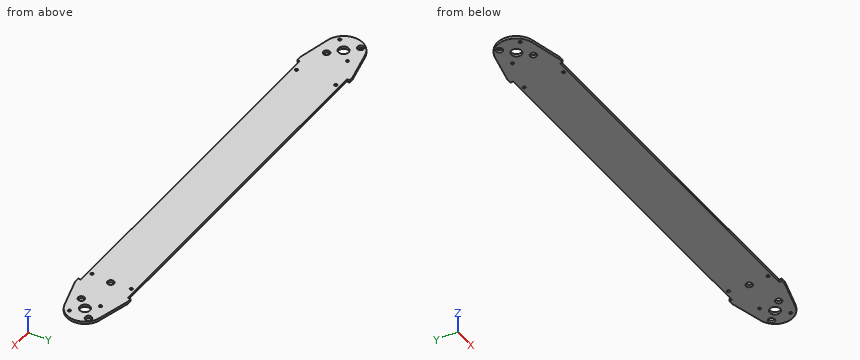
from build123d import *

# Parameters (mm, degrees)
F0_R     = 1.7272
F0_R_2   = 3.96875
F0_R_3   = 6.35
F1_DEPTH = 3.175


with BuildPart() as f1:
    # F0 (on Top) → F1 (new body)
    with BuildSketch(Plane.XY):
        with BuildLine():
            Line((-475.378193, 31.75), (-513.228467, 23.231407))
            ThreePointArc((-513.228467, 23.231407), (-531.812151, 0.128904), (-513.479674, -23.17344))
            Line((-513.479674, -23.17344), (-474.818103, -32.315493))
            Line((-474.818103, -32.315493), (-468.468103, -32.315493))
            Line((-468.468103, -32.315493), (-468.468103, -29.140493))
            Line((-468.468103, -29.140493), (-38.411718, -29.140493))
            Line((-38.411718, -29.140493), (-38.411718, -32.315493))
            Line((-38.411718, -32.315493), (-32.061718, -32.315493))
            Line((-32.061718, -32.315493), (6.126706, -21.36385))
            ThreePointArc((6.126706, -21.36385), (22.224151, 0.194294), (5.752253, 21.467701))
            Line((5.752253, 21.467701), (-32.621807, 31.75))
            Line((-32.621807, 31.75), (-38.971807, 31.75))
            Line((-38.971807, 31.75), (-38.971807, 28.575))
            Line((-38.971807, 28.575), (-469.028193, 28.575))
            Line((-469.028193, 28.575), (-469.028193, 31.75))
            Line((-469.028193, 31.75), (-475.378193, 31.75))
        make_face()
        with Locations((-454.180603, -24.377993)):
            Circle(F0_R, mode=Mode.SUBTRACT)
        with Locations((-520.909118, -12.909118)):
            Circle(F0_R, mode=Mode.SUBTRACT)
        with Locations((-495.090882, -12.909118)):
            Circle(F0_R_2, mode=Mode.SUBTRACT)
        with Locations((-52.699218, -24.377993)):
            Circle(F0_R, mode=Mode.SUBTRACT)
        with Locations((-11.786586, -11.786586)):
            Circle(F0_R_2, mode=Mode.SUBTRACT)
        with Locations((11.786586, -11.786586)):
            Circle(F0_R, mode=Mode.SUBTRACT)
        with Locations((-508, 0)):
            Circle(F0_R_3, mode=Mode.SUBTRACT)
        with Locations((-520.909118, 12.909118)):
            Circle(F0_R_2, mode=Mode.SUBTRACT)
        with Locations((-495.090882, 12.909118)):
            Circle(F0_R, mode=Mode.SUBTRACT)
        with Locations((-454.740693, 23.8125)):
            Circle(F0_R, mode=Mode.SUBTRACT)
        with Locations((-50.8, 0)):
            Circle(F0_R_2, mode=Mode.SUBTRACT)
        Circle(F0_R_3, mode=Mode.SUBTRACT)
        with Locations((-11.786586, 11.786586)):
            Circle(F0_R, mode=Mode.SUBTRACT)
        with Locations((11.786586, 11.786586)):
            Circle(F0_R_2, mode=Mode.SUBTRACT)
        with Locations((-53.259307, 23.8125)):
            Circle(F0_R, mode=Mode.SUBTRACT)
    extrude(amount=F1_DEPTH)


solid = f1.part
CAD build for the part. Positions are in the model's coordinates, mm. Give positions to 0.01 mm unless a question says otherwise; leave off trailing zeros. Order: outer loops, then holes, each group sorted by start corner. A loop starts at its lowest first (then second) coordinate and runs counter-clockwise, first axis right, second up. Notation, with made-up numbers: (11, 16) - (33, 16) arc R16 cw to (33, 35) - close; hole circle Ø10 at (-5.75, -33). An arc over 180 degrees is marked (long way). Write each question's results on one line, items separated by ' | '.
1. Saw through at C-C on x = -87.5. List the corners of the cut face in (y, z) (1 decimal).
Calculated:
outline: (-29.1, 0) - (28.6, 0) - (28.6, 3.2) - (-29.1, 3.2) - close
2. Probe L1, parallel to X at y = -15, z = 1.35; L2, parallel to X at y = -5, z = 2.2; L3, parallel to X at y = 11, z = 2.9. List the from-to ranges inside material, lowest first. Write a range as from..to.
Calculated:
L1: x = -526.49..-498.46, -491.72..-14.12, -9.46..16.4 | L2: x = -531.28..-511.91, -504.09..-3.91, 3.91..21.66 | L3: x = -529.12..-524.39, -517.43..-13.32, -10.25..7.9, 15.68..19.31
3. Saw through at B-B on z = 2.15. Count the separate pieces of the cut face and the enclosed holes in it, and give its area (3 significant figures).
Calculated:
separate pieces: 1 | enclosed holes: 15 | area: 30,400 mm2
4. Saw through at A-A on x = 0. List the corners of the cut face in (y, z) (3 decimals).
Calculated:
outline: (-23.121, 0) - (-6.35, 0) - (-6.35, 3.175) - (-23.121, 3.175) - close; (6.35, 0) - (23.009, 0) - (23.009, 3.175) - (6.35, 3.175) - close
5. Pin check, flat tips, straight feed: pin 1 (7 mm diameter, centred on x = 11.79, y = 11.79, fed in from +Z); pin 2 (1 mm diameter, centred on x = -232, z = 0.5, fed in from -Y); pin 3 (1 mm diameter, centred on x = -348.5, z = 0.5, fed in from +Y) (3 decimals). Stop position of each tip, or through.
Calculated:
pin 1: passes through | pin 2: stops at y = -29.14 | pin 3: stops at y = 28.575
